from build123d import *

# Parameters (mm, degrees)
F0_R     = 3.175
F1_DEPTH = 9.525
F2_SIZE2 = 1.4986
F2_SIZE  = 1.4986
F3_SIZE2 = 0.762
F3_SIZE  = 0.762
F5_DEPTH = 3.175


with BuildPart() as f1:
    # F0 (on Front) → F1 (new body)
    with BuildSketch(Plane.XZ):
        Circle(F0_R)
    extrude(amount=-F1_DEPTH)

    # F2
    f2_edges = [f1.edges().sort_by_distance(p)[0] for p in [
        (-3.175, 9.525, 0),
    ]]
    chamfer(f2_edges, length=F2_SIZE, length2=F2_SIZE2)

    # F3
    f3_edges = [f1.edges().sort_by_distance(p)[0] for p in [
        (-3.175, 0, 0),
    ]]
    chamfer(f3_edges, length=F3_SIZE, length2=F3_SIZE2)

    # F4 (on face) → F5 (cut)
    with BuildSketch(Plane.XZ):
        Polygon((0.916544, 1.5875), (-0.916544, 1.5875), (-1.833087, 0), (-0.916544, -1.5875), (0.916544, -1.5875), (1.833087, 0), align=None)
    extrude(amount=-F5_DEPTH, mode=Mode.SUBTRACT)


solid = f1.part
CAD build for the part. Positions are in the model's coordinates, mm. A direction names the side the tool comes from. Round coordinates to 2 decimals unless told otherwise and drop trailing zeros. Write each loop counter-clockwise with the first axis right and the second up, starting at its lowest first coordinate (ties: lowest second). Pieces come first, ordered by that corner, then holes. Notation, with made-up numbers: M 4,11.5 L 25,11.5 A22 ccw 25,42.5 Z; hole C -14.5,16.5 d10. An arc over 180 degrees is marked long. Put each result on its own line as item: value. Start each with the question number.
1) Saw through at C-C, the plane y = 7. Write the cut outline in (x, z) (3 decimals).
2) 3-axis set-ups, long thin cutter, end or side, ignore diameter. For faces 1 (the flat face through (0, 9.525, 0)), 2 (the flat face through (1.381, 1.565, 0.783)): which of +Z, -Z, +X, -X, +Y, -Y reach the whole face in a straight line?
3) Pull direction X, two halves, no side cores. Call faces 3 (the cylindrical face through (-0.69, 4.34, -3.1)), 4 (the flat face through (-1.37, 1.57, 0.8)), 5 (the flat face through (2, 0, 1)): pulls with the +X half, pulls with the -X half, needs draft (parallel to the pull), parting line crosses it, or undercut.
4) Saw through at B-B, the plane x = 0. Write the cut outline in (y, z) (1 decimal), and give its area (3 significant figures).
5) Saw through at D-D, the plane y = 8.5. Write the cut outline in (x, z), and give its area (3 significant figures).
6) Drill centre lines: probe 1 along Y at (x, z) = (-1.5, -0.25) (3 decimals); probe 2 along X at (y, z) = (1, 0.25); probe 3 along Z at (x, y) = (1.75, 1.5). Where is each one in solid material? Low to high. Write a range as [from, to].
7) Pin check, flat tip, straight feed: pin 1 Ø2 at (x, y) = (-2.5, 8.5) entering from +Z. Stop position of the tip, or through.
Resolved:
1. outline: C 0,0 d6.35
2. face 1: +Z, -Z, +X, -X, +Y
2. face 2: -Y
3. face 3: parting line crosses it
3. face 4: undercut
3. face 5: needs draft
4. outline: M 0,-2.4 L 0.8,-3.2 L 8,-3.2 L 9.5,-1.7 L 9.5,1.7 L 8,3.2 L 0.8,3.2 L 0,2.4 L 0,1.6 L 3.2,1.6 L 3.2,-1.6 L 0,-1.6 Z
4. area: 47.6 mm²
5. outline: C 0,0 d5.4
5. area: 22.9 mm²
6. probe 1: [3.175, 9.525]
6. probe 2: [-3.17, -1.69], [1.69, 3.17]
6. probe 3: [-2.65, -0.14], [0.14, 2.65]
7. pin 1: z = 2.73
